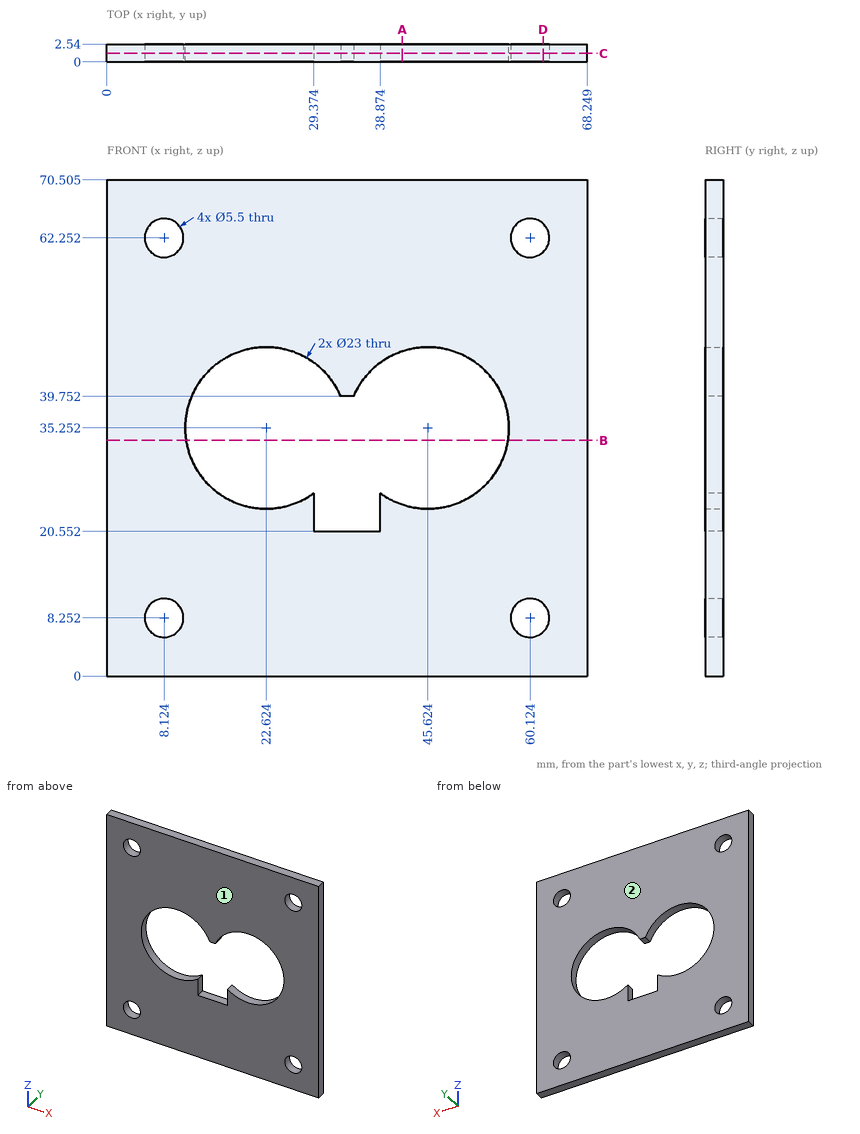
Here's the drawing with two shaded views (mm, measured from the low corner). I have some questions. Give positions to 0.01 mm unless a question says otherwise; leave off trailing zeros. Order: outer loops, then holes, each group sorted by start corner. A loop starts at its lowest first (then second) coordinate and runs counter-clockwise, first axis right, second up. Notation, with made-up numbers: (39, -16.75) -> (97, -16.75) arc R22 cw to (97, -5.75) -> close; hole circle Ø11 at (78.5, -10). An arc over 180 degrees is marked (long way). Use a Markdown table: item, result. Add a question column.
Item 1: I need wall thicknesses on line 1 (Z direction, x = 6, y = 0.5) (1 decimal); line 2 (X direction, y = 2.2, z = 40); line 3 (X direction, y = 2.45, z = 28). Which ranges of each line are inside material? Lowest first, please.
Item 2: Will this pin go through, and if not, where does the flat tip stop? pin 1 (1.3 mm diameter, centred on y = 1.5, z = 24, fed in from -X).
Item 3: Imagine slicing it at A-A on x = 42. Please give me the cut outline in (y, z) (1 decimal), plus the area to 3 significant figures.
Item 4: Imagine slicing it at D-D on x = 62. Please give me the cut outline in (y, z) (1 decimal).
Item 5: Imagine slicing it at C-C on y = 1.2. Give the number of separate pieces and of enclosed holes in the cut face, plus the area to 3 significant figures.
Item 6: Imagine slicing it at B-B on z = 33.5. Please give me the cut outline in (x, y).
Item 7: If we mould it in two halves opening along Y, with no side actions, what happens to the marked faces 1 and 2? For each: pulls with the +Y half, pulls with the -Y half, needs draft (parallel to the pull), parting line crosses it, or undercut.
Data:
| question | item | result |
|---|---|---|
| 1 | line 1 | z = 0 to 6.5, 10 to 60.5, 64 to 70.5 |
| 1 | line 2 | x = 0 to 12.15, 33.1 to 35.15, 56.1 to 68.25 |
| 1 | line 3 | x = 0 to 13.7, 54.55 to 68.25 |
| 2 | pin 1 | stops at x = 0 |
| 3 | outline | (0, 0) -> (2.5, 0) -> (2.5, 24.3) -> (0, 24.3) -> close; (0, 46.2) -> (2.5, 46.2) -> (2.5, 70.5) -> (0, 70.5) -> close |
| 3 | area | 124 mm² |
| 4 | outline | (0, 0) -> (2.5, 0) -> (2.5, 6.2) -> (0, 6.2) -> close; (0, 10.3) -> (2.5, 10.3) -> (2.5, 60.2) -> (0, 60.2) -> close; (0, 64.3) -> (2.5, 64.3) -> (2.5, 70.5) -> (0, 70.5) -> close |
| 5 | separate pieces | 1 |
| 5 | enclosed holes | 5 |
| 5 | area | 3,810 mm² |
| 6 | outline | (0, 0) -> (11.26, 0) -> (11.26, 2.54) -> (0, 2.54) -> close; (56.99, 0) -> (68.25, 0) -> (68.25, 2.54) -> (56.99, 2.54) -> close |
| 7 | face 1 | pulls with the -Y half |
| 7 | face 2 | pulls with the +Y half |
